Here's how the part is built. I have some questions about the finished solid (model axes, mm). Face numbers are marked on the shaded views. Round coordinates to 2 decimals unless told otherwise and drop trailing zeros. Order: outer loops, then holes, each group sorted by start corner. A loop starts at its lowest first (then second) coordinate and runs counter-clockwise, first axis right, second up. Notation, with made-up numbers: (60, -24.75) -> (88, -24.75) arc R13 ccw to (88, -18.75) -> close; hole circle Ø4 at (83, 60.25). An arc over 180 degrees is marked (long way). Answer in a Markdown table with one row per item.
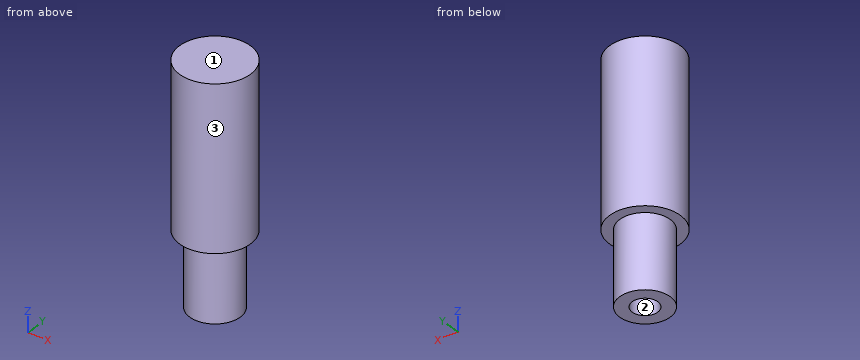
Autodesk Inventor part; units mm, degrees
ref_plane "YZ Plane" through (0, 0, 0) normal (1, 0, 0) x (0, 1, 0)
ref_plane "XZ Plane" through (0, 0, 0) normal (0, 1, 0) x (-1, 0, 0)
ref_plane "XY Plane" through (0, 0, 0) normal (0, 0, 1) x (1, 0, 0)
sketch "Sketch1" plane through (0, 0, 0) normal (0, 0, 1) x (1, 0, 0)
  circle A0 centre (0, 0) radius 6.6675
  circle A1 centre (0, 0) radius 4.7625
  dimension "d0" = 13.335
  dimension "d1" = 9.525
extrude "Extrusion1" add sketch "Sketch1" against normal blind 13.8684 contours A1
extrude "Extrusion2" add sketch "Sketch1" along normal blind 30.48 contours A0 | A1
thread "Thread1"
sketch "Sketch2" plane through (0, 0, -13.8684) normal (0, 0, -1) x (-1, 0, 0)
  circle A0 centre (0, 0) radius 4.7625
  circle A1 centre (0, 0) radius 2.413
  dimension "d8" = 4.826
extrude "Extrusion3" cut sketch "Sketch2" against normal blind 25.4 contours A1
thread "Thread2"
properties part number "Gear housing shaft BD drill motor"
1. Suppose I cut it at A-A on y = 0. Write out the boundary of the cut face in (x, z).
Numbers:
| item | result |
|---|---|
| outline | (-6.67, 0) -> (-4.76, 0) -> (-4.76, -13.87) -> (-2.41, -13.87) -> (-2.41, 11.53) -> (2.41, 11.53) -> (2.41, -13.87) -> (4.76, -13.87) -> (4.76, 0) -> (6.67, 0) -> (6.67, 30.48) -> (-6.67, 30.48) -> close |
2. Suppose I cut it at C-C on z = 8.5. Write out the boundary of the cut face in (x, y) (1 decimal).
Numbers:
| item | result |
|---|---|
| outline | circle Ø13.3 at (0, 0); hole circle Ø4.8 at (0, 0) |
3. Suppose I cut it at D-D on z = 17. Write out the boundary of the cut face in (x, y) (1 decimal), then the cut area to 3 significant figures.
Numbers:
| item | result |
|---|---|
| outline | circle Ø13.3 at (0, 0) |
| area | 140 mm2 |
4. We'd pull the mould along Y, two halves only. Please class the marked faces 1, 2 and 3: released by +Y, released by -Y, zero draft, split by the parting line, or undercut.
Numbers:
| item | result |
|---|---|
| face 1 | zero draft |
| face 2 | undercut |
| face 3 | split by the parting line |
5. Please list where these lines run through material, in increasing order: line 1 along Z through (x, y) = (-5.5, -2.25); line 2 along Y through (x, z) = (-0.25, 25); line 3 along Y through (x, z) = (0, 2.75).
Numbers:
| item | result |
|---|---|
| line 1 | z = 0 to 30.48 |
| line 2 | y = -6.66 to 6.66 |
| line 3 | y = -6.67 to -2.41, 2.41 to 6.67 |
6. For pin 1 Ø1.5 at (x, z) = (2.5, -0.5) entering from -Y; pin 2 Ø2 at (y, z) = (2, 16.5) entering from -X; pin 3 Ø6 at (x, z) = (1, 4) entering from -Y; pin 4 Ø2.5 at (x, y) = (1, 0) entering from -Z, each with a flat end and sliding along its axis, tell me the tip position at first contact or that it passes through.
Numbers:
| item | result |
|---|---|
| pin 1 | stops at y = -6.38 |
| pin 2 | stops at x = -6.59 |
| pin 3 | stops at y = -6.67 |
| pin 4 | stops at z = 11.53 |
